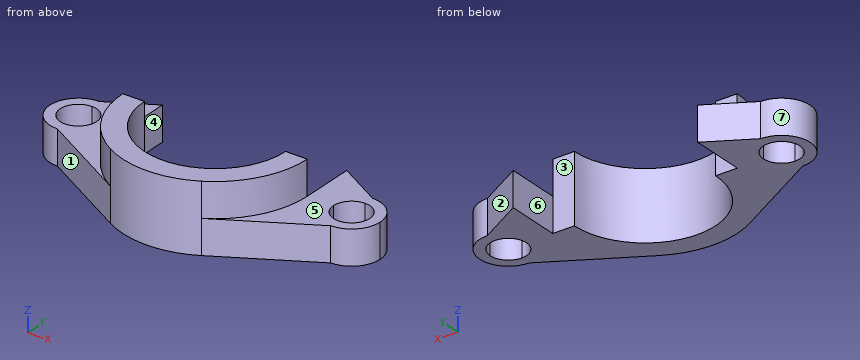
from build123d import *

# Parameters (mm, degrees)
F1_DEPTH = 6
F2_DEPTH = 3


with BuildPart() as f1:
    # F0 (on Top) → F1 (new body)
    with BuildSketch(Plane.XY):
        with BuildLine():
            Line((8.1, 0), (6.2, 0))
            ThreePointArc((6.2, 0), (0, -6.2), (-6.2, 0))
            Line((-6.2, 0), (-8.1, 0))
            ThreePointArc((-8.1, 0), (-7.0003956389, -4.074857163), (-4.0001331115, -7.0433610649))
            ThreePointArc((-4.0001331115, -7.0433610649), (0, -8.1), (4.0001331115, -7.0433610649))
            ThreePointArc((4.0001331115, -7.0433610649), (7.0003956389, -4.074857163), (8.1, 0))
        make_face()
    extrude(amount=F1_DEPTH)

    # F0 (on Top) → F2 (join)
    with BuildSketch(Plane.XY):
        with BuildLine():
            Line((9.5, 0), (8.1, 0))
            ThreePointArc((8.1, 0), (7.0003956389, -4.074857163), (4.0001331115, -7.0433610649))
            Line((4.0001331115, -7.0433610649), (12, -2.5))
            ThreePointArc((12, -2.5), (10.232233047, -1.767766953), (9.5, 0))
        make_face()
        with BuildLine():
            Line((10.4, 0), (9.5, 0))
            ThreePointArc((9.5, 0), (10.232233047, -1.767766953), (12, -2.5))
            Line((12, -2.5), (12, -1.6))
            ThreePointArc((12, -1.6), (10.8686291501, -1.1313708499), (10.4, 0))
        make_face()
        with BuildLine():
            Line((12, -1.6), (12, -2.5))
            ThreePointArc((12, -2.5), (13.767766953, -1.767766953), (14.5, 0))
            ThreePointArc((14.5, 0), (13.767766953, 1.767766953), (12, 2.5))
            Line((12, 2.5), (12, 1.6))
            ThreePointArc((12, 1.6), (13.1313708499, 1.1313708499), (13.6, 0))
            ThreePointArc((13.6, 0), (13.1313708499, -1.1313708499), (12, -1.6))
        make_face()
        with BuildLine():
            ThreePointArc((-4.0001331115, -7.0433610649), (-7.0003956389, -4.074857163), (-8.1, 0))
            Line((-8.1, 0), (-9.5, 0))
            ThreePointArc((-9.5, 0), (-10.232233047, -1.767766953), (-12, -2.5))
            Line((-12, -2.5), (-4.0001331115, -7.0433610649))
        make_face()
        with BuildLine():
            ThreePointArc((12, 2.5), (10.232233047, 1.767766953), (9.5, 0))
            Line((9.5, 0), (10.4, 0))
            ThreePointArc((10.4, 0), (10.8686291501, 1.1313708499), (12, 1.6))
            Line((12, 1.6), (12, 2.5))
        make_face()
        with BuildLine():
            ThreePointArc((-12, -2.5), (-10.232233047, -1.767766953), (-9.5, 0))
            Line((-9.5, 0), (-10.4, 0))
            ThreePointArc((-10.4, 0), (-10.8686291501, -1.1313708499), (-12, -1.6))
            Line((-12, -1.6), (-12, -2.5))
        make_face()
        with BuildLine():
            ThreePointArc((-12, 2.5), (-14.5, 0), (-12, -2.5))
            Line((-12, -2.5), (-12, -1.6))
            ThreePointArc((-12, -1.6), (-13.6, 0), (-12, 1.6))
            Line((-12, 1.6), (-12, 2.5))
        make_face()
        with BuildLine():
            Line((-10.4, 0), (-9.5, 0))
            ThreePointArc((-9.5, 0), (-10.232233047, 1.767766953), (-12, 2.5))
            Line((-12, 2.5), (-12, 1.6))
            ThreePointArc((-12, 1.6), (-10.8686291501, 1.1313708499), (-10.4, 0))
        make_face()
        with BuildLine():
            Line((-9.5, 0), (-8.1, 0))
            Line((-8.1, 0), (-8.1, 4.7149253731))
            Line((-8.1, 4.7149253731), (-12, 2.5))
            ThreePointArc((-12, 2.5), (-10.232233047, 1.767766953), (-9.5, 0))
        make_face()
        with BuildLine():
            Line((8.1, 4.7149253731), (8.1, 0))
            Line((8.1, 0), (9.5, 0))
            ThreePointArc((9.5, 0), (10.232233047, 1.767766953), (12, 2.5))
            Line((12, 2.5), (8.1, 4.7149253731))
        make_face()
    extrude(amount=F2_DEPTH)


solid = f1.part
The model under review builds one solid part; all positions refer to its coordinate system, in mm. Face numbers are marked on the shaded views. A direction names the side the tool comes from. Coordinates: 2 decimals unless noted, no trailing zeros. Write each loop counter-clockwise with the first axis right and the second up, starting at its lowest first coordinate (ties: lowest second). Pieces come first, ordered by that corner, then holes. Notation, with made-up numbers: M 42,-32.5 L 71,-32.5 A22 cw 71,-2.5 Z; hole C -13,0.25 d9. An arc over 180 degrees is marked long. Put each result on its own line as item: value.
1) Clearance check with flat-ended pins moving along their axes: pin 1 Ø3.5 at (y, z) = (3.5, 1.5) entering from +X; pin 2 Ø1.5 at (x, y) = (9, -1) entering from +Z; pin 3 Ø1 at (y, z) = (-2.5, 5.5) entering from +X. State where each tip first meets the part, or that it passes through.
Computed:
pin 1: stops at x = 13.79
pin 2: stops at z = 3
pin 3: stops at x = 7.85
2) Add section D-D on x = 0. Give the boundary of the cut face in (y, z), then the cut area to 3 significant figures.
Computed:
outline: M -8.1,0 L -6.2,0 L -6.2,6 L -8.1,6 Z
area: 11.4 mm2
3) Add section C-C on z = 3.45. Give the boundary of the cut face in (x, y), then the cut area to 3 significant figures.
Computed:
outline: M -8.1,0 A8.1 ccw 8.1,0 L 6.2,0 A6.2 cw -6.2,0 Z
area: 42.7 mm2
4) Draft analysis for pull direction X (two halves, no side actions). For the marked faces 1, 2, 3 and 4, state which applies: released by +X, released by -X, zero draft, split by the parting line, or undercut.
Computed:
face 1: released by -X
face 2: released by +X
face 3: undercut
face 4: undercut
5) For the marked faces 5, 6 and 7, list the 3-axis set-ups (+Z, -Z, +X, -X, +Y, -Y) from which the entire face can be reached by the end or side of a thin tool; tool diameter is ignored.
Computed:
face 5: +Z, +X, -Y
face 6: +Z, -Z, +Y
face 7: +Z, -Z, -X
6) Add section B-B on y = -5.25. Give the boundary of the cut face in (x, z), then the cut area to 3 significant figures.
Computed:
outline: M -7.16,0 L -3.3,0 L -3.3,6 L -6.17,6 L -6.17,3 L -7.16,3 Z; M 3.3,0 L 7.16,0 L 7.16,3 L 6.17,3 L 6.17,6 L 3.3,6 Z
area: 40.4 mm2
7) Wall thickness on probe 1 along X at (y, z) = (0.75, 0.75); probe 2 along Z at (x, y) = (-8.75, 1.25); probe 3 along X at (y, z) = (-1.5, 3.25): over which ranges is each line inside the solid? List them lowest first. Write a range as [from, to].
Computed:
probe 1: x = [-14.38, -13.41], [-10.59, -8.1], [8.1, 10.59], [13.41, 14.38]
probe 2: z = [0, 3]
probe 3: x = [-7.96, -6.02], [6.02, 7.96]
8) Add section A-A on z = 0.4. Give the boundary of the cut face in (x, y).
Computed:
outline: M -12,-2.5 L -4,-7.04 A8.1 ccw 4,-7.04 L 12,-2.5 A2.5 ccw 12,2.5 L 8.1,4.71 L 8.1,0 L 6.2,0 A6.2 cw -6.2,0 L -8.1,0 L -8.1,4.71 L -12,2.5 A2.5 ccw Z; hole C -12,0 d3.2; hole C 12,0 d3.2
